```python
from build123d import *

# Parameters (mm, degrees)
F0_W     = 10.5
F0_H     = 27.5
F1_DEPTH = 40
F3_DEPTH = 120.3
F4_W     = 17.5
F4_H     = 17
F5_DEPTH = 2.5
F6_R     = 2


with BuildPart() as f1:
    # F0 (on Top) → F1 (new body)
    with BuildSketch(Plane.XY):
        with Locations((-49.75, -13.75)):
            Rectangle(F0_W, F0_H)
        with BuildLine():
            Line((55, 0), (55, 27.5))
            Line((55, 27.5), (-55, 27.5))
            Line((-55, 27.5), (-55, 0))
            Line((-55, 0), (-44.5, 0))
            ThreePointArc((-44.5, 0), (-27.5, 17), (-10.5, 0))
            Line((-10.5, 0), (0, 0))
            Line((0, 0), (10.5, 0))
            ThreePointArc((10.5, 0), (27.5, 17), (44.5, 0))
            Line((44.5, 0), (55, 0))
        make_face()
        Polygon((10.5, -27.5), (10.5, 0), (0, 0), (-10.5, 0), (-10.5, -27.5), align=None)
        with Locations((49.75, -13.75)):
            Rectangle(F0_W, F0_H)
    extrude(amount=F1_DEPTH)

    # F2 (on face) → F3 (cut)
    with BuildSketch(Plane(origin=(-55, 0, 0), x_dir=(0, -1, 0), z_dir=(-1, 0, 0))):
        with BuildLine():
            add(Edge.make_bspline(
                [(27.5, 37), (-22.500001, 37), (-22.500001, 0)],
                knots=[4.712389, 4.712389, 4.712389, 6.283185, 6.283185, 6.283185], degree=2, weights=[1, 0.707107, 1]))
            Line((-22.500001, 0), (27.5, 0))
            Line((27.5, 0), (27.5, 37))
        make_face()
    extrude(amount=-F3_DEPTH, mode=Mode.SUBTRACT)

    # F4 (on face) → F5 (cut)
    with BuildSketch(Plane(origin=(0, 27.5, 0), x_dir=(-1, 0, 0), z_dir=(0, 1, 0))):
        with Locations((-36.25, 30)):
            Rectangle(F4_W, F4_H)
        with Locations((-18.75, 30)):
            Rectangle(F4_W, F4_H)
        with Locations((16.651222, 30)):
            Rectangle(F4_W, F4_H)
        with Locations((34.151222, 30)):
            Rectangle(F4_W, F4_H)
    extrude(amount=-F5_DEPTH, mode=Mode.SUBTRACT)

    # F6
    f6_edges = [f1.edges().sort_by_distance(p)[0] for p in [
        (-44.5, -13.75, 40),
        (10.5, -13.75, 40),
        (55, 0, 40),
        (-55, 0, 40),
    ]]
    fillet(f6_edges, radius=F6_R)


solid = f1.part
```
Here's how the part is built. I have some questions about the finished solid (model axes, mm). A direction names the side the tool comes from. Round coordinates to 2 decimals unless told otherwise and drop trailing zeros. Use a Markdown table: item, result. Add a question column.
(1) I need wall thicknesses on line 1 along X through (y, z) = (-14, 37); line 2 along X through (y, z) = (5, 30); line 3 along Y through (x, z) = (-27.5, 22.5). Which ranges of each line are inside material? Lowest first, please.
(2) For faces 4 (the face through (44.5, -8, 36)), 5 (the face through (45, 26, 30)), 6 (the face through (55, 14, 26)), which set-ups out of +Z, -Z, +X, -X, +Y, -Y let a thin tool reach every point of the face, with its end or its side?
(3) If we mould it in two halves opening along Z, with no side actions, what happens to faces 1 (the face through (-25, 26, 21.5)), 2 (the face through (45.1, -13.94, 39.43)), 3 (the face through (-44.5, -8, 36))? For each: released by +Z, released by -Z, zero draft, split by the parting line, or undercut.
(4) For pin 1 Ø2 at (x, y) = (0, 0) entering from -Z; pin 2 Ø8.5 at (x, z) = (-27.5, 33) entering from +Y, each with a flat end and sliding along its axis, tell me the tip position at first contact or that it passes through.
(5) Suppose I cut it at A-A, the plane y = -20. Count the separate pieces of the cut face and the enclosed holes in it, and give its area (3 significant figures).
Verdict:
| question | item | result |
|---|---|---|
| 1 | line 1 | -55 to -44.5, -10.5 to 10.5, 44.5 to 55 |
| 1 | line 2 | -55 to -43.75, -11.25 to 11.25, 43.75 to 55 |
| 1 | line 3 | 17 to 25 |
| 2 | face 4 | +Z, -Z, -Y |
| 2 | face 5 | +Y |
| 2 | face 6 | +Z, -Z, +X, +Y, -Y |
| 3 | face 1 | undercut |
| 3 | face 2 | released by +Z |
| 3 | face 3 | zero draft |
| 4 | pin 1 | z = 30.4 |
| 4 | pin 2 | y = 25 |
| 5 | separate pieces | 3 |
| 5 | enclosed holes | 0 |
| 5 | area | 138 mm2 |
